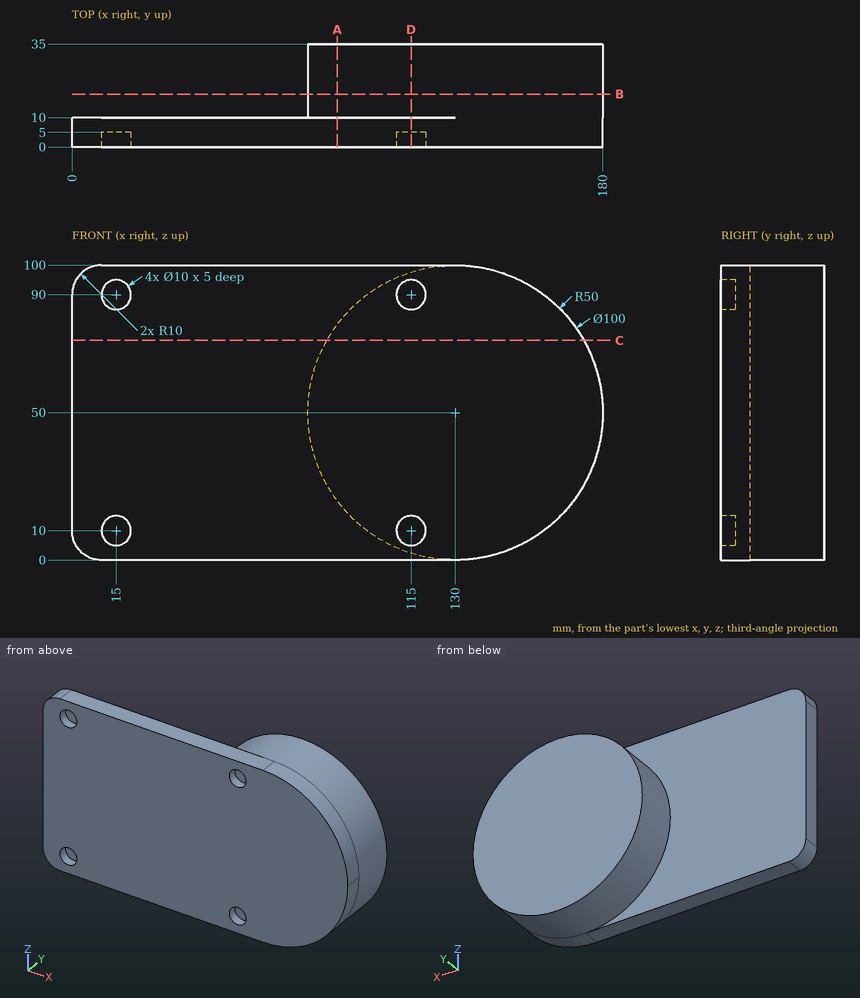
Design review of the part shown in the three views and the two pictorial views. Dimensions are in mm from the part's minimum x, y and z. Round coordinates to 2 decimals unless told otherwise and drop trailing zeros. Order: outer loops, then holes, each group sorted by start corner. A loop starts at its lowest first (then second) coordinate and runs counter-clockwise, first axis right, second up.
Q1. We need section B-B, the plane y = 18. Give the boundary of the cut face in (x, z).
Findings below:
outline: circle Ø100 at (130, 50)
Q2. Wall thickness on line 1 (X direction, y = 3, z = 9.5); line 2 (Y direction, x = 37, z = 75); line 3 (X direction, y = 18, z = 34.5): over which ranges is each line inside the solid? List them lowest first.
Findings below:
line 1: x = 0.01 to 10.03, 19.97 to 110.03, 119.97 to 159.32
line 2: y = 0 to 10
line 3: x = 82.46 to 177.54
Q3. Insertion check: P1, Ø9, axis at x = 15, z = 10, coming from the +Y side; P2, Ø4, axis at x = 72, y = 11.5, coming from the -Z side; P3, Ø1.5, axis at y = 28.5, z = 58, coming from the +X side; P4, Ø8, axis at y = 15.5, z = 45.5, coming from the -X side. Each pin has a flat end and moves straight along its axis. Give the tip position at first contact, or say it passes through.
Findings below:
P1: stops at y = 10
P2: stops at z = 0
P3: stops at x = 179.47
P4: stops at x = 80
Q4. We need section A-A, the plane x = 90. Give the boundary of the cut face in (y, z).
Findings below:
outline: (0, 0) - (10, 0) - (10, 20) - (35, 20) - (35, 80) - (10, 80) - (10, 100) - (0, 100) - close
Q5. We need section C-C, the plane z = 74.5. Give the boundary of the cut face in (x, y), plus the area to 3 significant figures.
Findings below:
outline: (0, 0) - (173.59, 0) - (173.59, 35) - (86.41, 35) - (86.41, 10) - (0, 10) - close
area: 3,920 mm2
Q6. We need section D-D, the plane x = 115. Give the boundary of the cut face in (y, z).
Findings below:
outline: (0, 0) - (10, 0) - (10, 2.3) - (35, 2.3) - (35, 97.7) - (10, 97.7) - (10, 100) - (0, 100) - (0, 95) - (5, 95) - (5, 85) - (0, 85) - (0, 15) - (5, 15) - (5, 5) - (0, 5) - close
